Autodesk Inventor part; units mm, degrees
ref_plane "YZ Plane" through (0, 0, 0) normal (1, 0, 0) x (0, 1, 0)
ref_plane "XZ Plane" through (0, 0, 0) normal (0, 1, 0) x (-1, 0, 0)
ref_plane "XY Plane" through (0, 0, 0) normal (0, 0, 1) x (1, 0, 0)
sketch "Boceto1" plane through (0, 0, 0) normal (0, 0, 1) x (1, 0, 0)
  circle A0 centre (-24.75, 100) radius 51.4081
  circle A1 centre (-24.75, 100) radius 70
  point P0 (0, 0)
  dimension "d0" = 140
extrude "Extrusión1" add sketch "Boceto1" along normal blind 3 contours A0 | A1
sketch "Boceto2" plane through (-24.75, 100, 0) normal (0, 0, -1) x (-1, 0, 0)
  circle A0 centre (0, 0) radius 6.4
  point P0 (-24.75, -100)
  dimension "d3" = 12.8
extrude "Extrusión2" add sketch "Boceto2" along normal blind 10
sketch "Boceto3" plane through (-24.75, 100, -10) normal (0, 0, -1) x (-1, 0, 0)
  circle A0 centre (0, 0) radius 6.4
  point P0 (-24.75, -100)
hole "Agujero1" at (-24.75, 100, -10) direction (0, 0, 1) diameter 5.6 depth 4
fillet "Empalme1" radius 3 1 edges at (-18.35, 100, 0)
properties part number "Base_Plato"
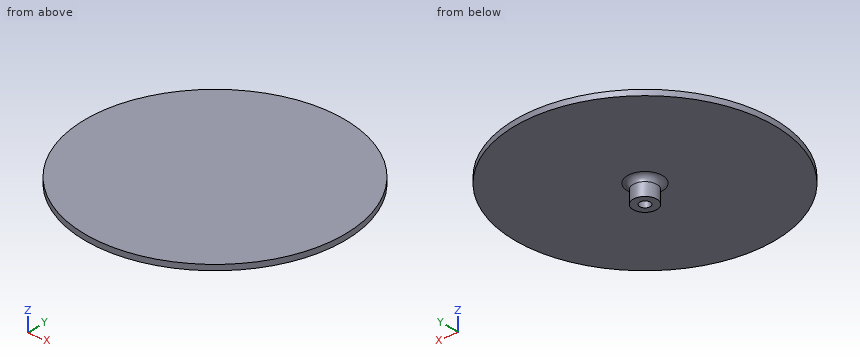
Here's how the part is built. I have some questions about the finished solid (model axes, mm). Round coordinates to 2 decimals unless told otherwise and drop trailing zeros. Order: outer loops, then holes, each group sorted by start corner. A loop starts at its lowest first (then second) coordinate and runs counter-clockwise, first axis right, second up. Notation, with made-up numbers: M -12.75,6.25 L 34.25,6.25 A26 ccw 34.25,20.25 Z; hole C -35,-9 d3. An arc over 180 degrees is marked long. One line per question, with ' | ' between items.
1) I'm going to push flat-ended pins straight in: pin 1 Ø3 at (x, z) = (-26.5, -8.5) entering from -Y; pin 2 Ø5 at (x, z) = (-32.5, 1.5) entering from -Y; pin 3 Ø2 at (x, z) = (-77, -2) entering from -Y. Where does each tip first touch, or does it pass through?
Checked values:
pin 1: stops at y = 93.6 | pin 2: stops at y = 30.2 | pin 3: passes through
2) Imagine slicing it at B-B, the plane x = -24.75. Write out the boundary of the cut face in (y, z), plus the area to 3 significant figures.
Checked values:
outline: M 30,0 L 90.6,0 A3 cw 93.6,-3 L 93.6,-10 L 97.2,-10 L 97.2,-6 L 102.8,-6 L 102.8,-10 L 106.4,-10 L 106.4,-3 A3 cw 109.4,0 L 170,0 L 170,3 L 30,3 Z | area: 529 mm²
3) Imagine slicing it at C-C, the plane y = 149. Write out the boundary of the cut face in (x, z), plus the area to 3 significant figures.
Checked values:
outline: M -74.74,0 L 25.24,0 L 25.24,3 L -74.74,3 Z | area: 300 mm²
4) I need wall thicknesses on line 1 (Y direction, x = -24.75, z = -6.85); line 2 (Z direction, x = -32.5, y = 48.5); line 3 (X direction, y = 120.5, z = 2.5). Which ranges of each line are inside material? Lowest first, please.
Checked values:
line 1: y = 93.6 to 97.2, 102.8 to 106.4 | line 2: z = 0 to 3 | line 3: x = -91.68 to 42.18
5) Imagine slicing it at D-D, the plane x = -8.5. Write out the boundary of the cut face in (y, z).
Checked values:
outline: M 31.91,0 L 168.09,0 L 168.09,3 L 31.91,3 Z
6) Imagine slicing it at A-A, the plane y = 100. Write out the boundary of the cut face in (x, z), plus the area to 3 significant figures.
Checked values:
outline: M -94.75,0 L -34.15,0 A3 cw -31.15,-3 L -31.15,-10 L -27.55,-10 L -27.55,-6 L -21.95,-6 L -21.95,-10 L -18.35,-10 L -18.35,-3 A3 cw -15.35,0 L 45.25,0 L 45.25,3 L -94.75,3 Z | area: 529 mm²
